from build123d import *

# Parameters (mm, degrees)
ESQUISSE1_R             = 45
BOSS_EXTRU_1_DEPTH      = 30
ESQUISSE2_R             = 25
BOSS_EXTRU_2_DEPTH      = 40
ESQUISSE3_R             = 5
ENL_V_MAT_EXTRU_1_DEPTH = 71
ESQUISSE6_R             = 5
ENL_V_MAT_EXTRU_3_DEPTH = 10
ESQUISSE7_R             = 5
ENL_V_MAT_EXTRU_4_DEPTH = 10


with BuildPart() as part:
    # Esquisse1 → Boss.-Extru.1 (new body)
    with BuildSketch(Plane.XY):
        Circle(ESQUISSE1_R)
    extrude(amount=BOSS_EXTRU_1_DEPTH)

    # Esquisse2 → Boss.-Extru.2 (add)
    with BuildSketch(Plane.XY.offset(30)):
        Circle(ESQUISSE2_R)
    extrude(amount=BOSS_EXTRU_2_DEPTH)

    # Esquisse3 → Enlèv. mat.-Extru.1 (cut, through all)
    with BuildSketch(Plane.XY.offset(70)):
        Circle(ESQUISSE3_R)
    extrude(amount=-ENL_V_MAT_EXTRU_1_DEPTH, mode=Mode.SUBTRACT)

    # Esquisse6 → Enlèv. mat.-Extru.3 (cut)
    with BuildSketch(Plane.XY.offset(70)):
        with Locations((0, 15)):
            Circle(ESQUISSE6_R)
    extrude(amount=-ENL_V_MAT_EXTRU_3_DEPTH, mode=Mode.SUBTRACT)

    # Esquisse7 → Enlèv. mat.-Extru.4 (cut)
    with BuildSketch(Plane(origin=(0, 0, 0), x_dir=(-1, 0, 0), z_dir=(0, 0, -1))):
        with Locations((0, 15)):
            Circle(ESQUISSE7_R)
    extrude(amount=-ENL_V_MAT_EXTRU_4_DEPTH, mode=Mode.SUBTRACT)


solid = part.part
Source: CAD feature listing. Evaluate the final solid. Frame: model axes, mm. A direction names the side the tool comes from. Give positions to 0.01 mm unless a question says otherwise; leave off trailing zeros. Loops run counter-clockwise (first coordinate to the right, second up) from the corner with the lowest first, then second, coordinate; pieces in that order, holes last. Notation, with made-up numbers: (11.5, 81) -> (31.5, 81) arc R21 cw to (31.5, 99) -> close; hole circle Ø3 at (56.5, 77.5). An arc over 180 degrees is marked (long way). Use a Markdown table: item, result. Add a question column.
1) Line query: line 1 along Y through (x, z) = (0, 5.25); line 2 along Y through (x, z) = (0, 64); line 3 along Y through (x, z) = (0, 26). Output: solid intervals per line, ascending. Write a range as [from, to].
2) First-contact query: pin 1 (3 mm diameter, centred on x = 9.5, z = 57, fed in from -Y); pin 2 (10 mm diameter, centred on y = 10.5, z = 60, fed in from +X); pin 3 (3 mm diameter, centred on x = 28.5, y = 22.5, fed in from +Z). Flat tips, straight axial feed; report the tip coordinate or a pass-through.
3) Pull-direction query (Y, two-part tool) for faces 4 (the face through (-1.08, -4.88, 35.49)), 5 (the face through (23.846, 7.509, 49.72)), 6 (the face through (19, -19, 30)); classes: +Y half, -Y half, draft (parallel to the pull), parting line (faces both ways), or undercut.
4) Section query B-B, the plane x = 0. Return the cut outline in (y, z), then the cut area to 3 significant figures.
5) Reachability of faces 1 (the face through (0, 15, 10)), 2 (the face through (-0.3, -5.2, 70)), 3 (the face through (0, 15, 60)) from +Z, -Z, +X, -X, +Y, -Y: full face, straight path, thin tool, end or side. Return the list, or none.
6) Section query D-D, the plane x = -14. Return the cut outline in (y, z).
7) Section query C-C, the plane z = 49. Return the cut outline in (x, y), then the cut area to 3 significant figures.
8) Section query A-A, the plane y = 0. Return the cut outline in (x, z), then the cut area to 3 significant figures.
Numbers:
| question | item | result |
|---|---|---|
| 1 | line 1 | y = [-45, -5], [5, 10], [20, 45] |
| 1 | line 2 | y = [-25, -5], [5, 10], [20, 25] |
| 1 | line 3 | y = [-45, -5], [5, 45] |
| 2 | pin 1 | stops at y = -23.69 |
| 2 | pin 2 | stops at x = 24.39 |
| 2 | pin 3 | stops at z = 30 |
| 3 | face 4 | undercut |
| 3 | face 5 | parting line |
| 3 | face 6 | draft |
| 4 | outline | (-45, 0) -> (-5, 0) -> (-5, 70) -> (-25, 70) -> (-25, 30) -> (-45, 30) -> close; (5, 0) -> (10, 0) -> (10, 10) -> (20, 10) -> (20, 0) -> (45, 0) -> (45, 30) -> (25, 30) -> (25, 70) -> (20, 70) -> (20, 60) -> (10, 60) -> (10, 70) -> (5, 70) -> close |
| 4 | area | 3,800 mm2 |
| 5 | face 1 | -Z |
| 5 | face 2 | +Z, +X, -X, +Y, -Y |
| 5 | face 3 | +Z |
| 6 | outline | (-42.77, 0) -> (42.77, 0) -> (42.77, 30) -> (20.71, 30) -> (20.71, 70) -> (-20.71, 70) -> (-20.71, 30) -> (-42.77, 30) -> close |
| 7 | outline | circle Ø50 at (0, 0); hole circle Ø10 at (0, 0) |
| 7 | area | 1,880 mm2 |
| 8 | outline | (-45, 0) -> (-5, 0) -> (-5, 70) -> (-25, 70) -> (-25, 30) -> (-45, 30) -> close; (5, 0) -> (45, 0) -> (45, 30) -> (25, 30) -> (25, 70) -> (5, 70) -> close |
| 8 | area | 4,000 mm2 |
